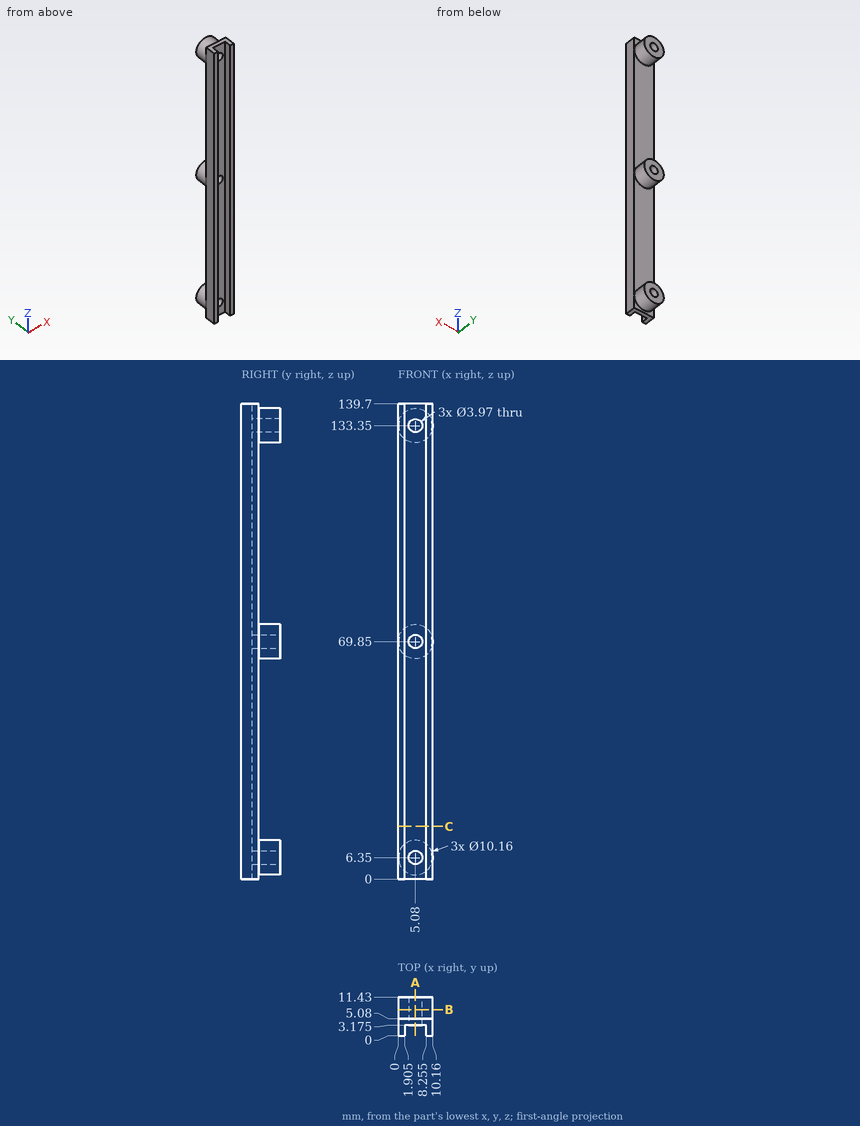
Geometry check sheet. Reference: drawing and pictorial views, mm from the part's lowest x, y, z. Give positions to 0.01 mm unless a question says otherwise; leave off trailing zeros. Write each loop counter-clockwise with the first axis right and the second up, starting at its lowest first coordinate (ties: lowest second). Pieces come first, ordered by that corner, then holes. Notation, with made-up numbers: (-37, 4) - (-25, 4) arc R19 cw to (-25, 27) - close; hole circle Ø3 at (3.5, 57). An arc over 180 degrees is marked (long way). Use a Markdown table: item, result.
Q1. Section check C-C, the plane z = 15.5. Enter the section's corners in (x, y) (3 decimals), then the cut area to 3 significant figures.
Computed:
| item | result |
|---|---|
| outline | (0, 0) - (1.905, 0) - (1.905, 3.175) - (8.255, 3.175) - (8.255, 0) - (10.16, 0) - (10.16, 5.08) - (0, 5.08) - close |
| area | 31.5 mm² |
Q2. Section check A-A, the plane x = 5.08. Enter the section's corners in (y, z) (3 decimals).
Computed:
| item | result |
|---|---|
| outline | (3.175, 0) - (5.08, 0) - (5.08, 1.27) - (11.43, 1.27) - (11.43, 4.365) - (3.175, 4.365) - close; (3.175, 8.335) - (11.43, 8.335) - (11.43, 11.43) - (5.08, 11.43) - (5.08, 64.77) - (11.43, 64.77) - (11.43, 67.865) - (3.175, 67.865) - close; (3.175, 71.835) - (11.43, 71.835) - (11.43, 74.93) - (5.08, 74.93) - (5.08, 128.27) - (11.43, 128.27) - (11.43, 131.365) - (3.175, 131.365) - close; (3.175, 135.335) - (11.43, 135.335) - (11.43, 138.43) - (5.08, 138.43) - (5.08, 139.7) - (3.175, 139.7) - close |
Q3. Section check B-B, the plane y = 7.75. Enter the section's corners in (x, z) (3 decimals).
Computed:
| item | result |
|---|---|
| outline | circle Ø10.16 at (5.08, 6.35); circle Ø10.16 at (5.08, 69.85); circle Ø10.16 at (5.08, 133.35); hole circle Ø3.97 at (5.08, 6.35); hole circle Ø3.97 at (5.08, 69.85); hole circle Ø3.97 at (5.08, 133.35) |
Q4. Thickness scan on L1, parallel to Z at x = 5.08, y = 7.25 (3 decimals); L2, parallel to X at y = 8.5, z = 69.85 (3 decimals); L3, parallel to Z at x = 6, y = 10.5. Record the ranges inside material, lowest first. Write a range as [from, to].
Computed:
| item | result |
|---|---|
| L1 | z = [1.27, 4.365], [8.335, 11.43], [64.77, 67.865], [71.835, 74.93], [128.27, 131.365], [135.335, 138.43] |
| L2 | x = [0, 3.095], [7.065, 10.16] |
| L3 | z = [1.35, 4.59], [8.11, 11.35], [64.85, 68.09], [71.61, 74.85], [128.35, 131.59], [135.11, 138.35] |
Q5. Go/stop test with flat-tipped pins: P1, Ø6, axis at x = 4.5, y = 9, coming from the +Z side; P2, Ø3, axis at x = 7, z = 37.5, coming from the +Y side; P3, Ø1.5, axis at x = 4.5, z = 26.5, coming from the -Y side (3 decimals). Record where each tip stops, or that it passes through.
Computed:
| item | result |
|---|---|
| P1 | stops at z = 138.43 |
| P2 | stops at y = 5.08 |
| P3 | stops at y = 3.175 |
